from build123d import *

# Parameters (mm, degrees)
F0_W     = 50.8
F0_H     = 38.1
F1_DEPTH = 31.75
F3_DEPTH = 50.8
F4_W     = 18.9170949161
F4_H     = 6.0472670011
F4_W_2   = 4.9618594348
F5_DEPTH = 19.05
F6_DEPTH = 25.4


with BuildPart() as f1:
    # F0 (on Front) → F1 (new body)
    with BuildSketch(Plane.XZ):
        with Locations((-6.0472674668, 14.0159087854)):
            Rectangle(F0_W, F0_H)
    extrude(amount=F1_DEPTH)

    # F2 (on face) → F3 (cut)
    with BuildSketch(Plane.YZ.offset(19.3527325332)):
        with BuildLine():
            Line((-31.75, 33.0659087854), (-31.75, 6.0472674668))
            ThreePointArc((-31.75, 6.0472674668), (-11.6942038752, 12.7030410182), (-6.0472670011, 33.0659087854))
            Line((-6.0472670011, 33.0659087854), (-31.75, 33.0659087854))
        make_face()
    extrude(amount=-F3_DEPTH, mode=Mode.SUBTRACT)

    # F4 (on face) → F5 (cut)
    with BuildSketch(Plane.XY.offset(33.0659087854)):
        with Locations((-3.4112781286, -3.0236335006)):
            Rectangle(F4_W, F4_H)
        with Locations((-15.3507553041, -3.0236335006)):
            Rectangle(F4_W_2, F4_H)
    extrude(amount=-F5_DEPTH, mode=Mode.SUBTRACT)

    # F6 (cut): a face of the model
    f6_faces = [f1.faces().sort_by_distance(p)[0] for p in [
        (-5.892207846, -6.0472670011, 18.653876051),
    ]]
    extrude(f6_faces, amount=-F6_DEPTH, mode=Mode.SUBTRACT)


solid = f1.part
Can you work these out from the model? Positions are in its coordinate system, mm. A direction names the side the tool comes from. Coordinates: 2 decimals unless noted, no trailing zeros. Write each loop counter-clockwise with the first axis right and the second up, starting at its lowest first coordinate (ties: lowest second). Pieces come first, ordered by that corner, then holes. Notation, with made-up numbers: M 68.5,41 L 82.5,41 A29 ccw 82.5,72 Z; hole C -23,16.5 d5. An arc over 180 degrees is marked long. Use one line per item in the form item = value.
Q1. If we section it at A-A (z = 28): Write out the boundary of the cut face in (x, y).
Model answer:
outline = M -31.45,-5.51 L -17.83,-5.51 L -17.83,0 L -31.45,0 Z; M 6.05,-5.51 L 19.35,-5.51 L 19.35,0 L 6.05,0 Z
Q2. We'd pull the mould along X, two halves only. Please class faces 3 (the flat face through (-31.447, -12, 5)), 4 (the flat face through (-17.832, -3, 24)), 5 (the flat face through (19.353, -12, 5)), 6 (the flat face through (-6, -5, 14.016)): +X half, -X half, draft (parallel to the pull), parting line (faces both ways), or undercut.
Model answer:
face_3 = -X half
face_4 = undercut
face_5 = +X half
face_6 = undercut
Q3. For faces 1 (the flat face through (-6, 0, 10)), 2 (the flat face through (6.047, -3, 24)), which set-ups out of +Z, -Z, +X, -X, +Y, -Y let a thin tool reach every point of the face, with its end or its side?
Model answer:
face_1 = +Z, -Z, +X, -X, +Y
face_2 = +Z, +Y, -Y
Q4. I need wall thicknesses on line 1 along X through (y, z) = (-6.5, 17.5); line 2 along Z through (x, y) = (-13, -7); line 3 along Z through (x, y) = (6, -27). Which ranges of each line are inside material? Lowest first, please. Write a range as from..to.
Model answer:
line_1 = -31.45..-17.83, 6.05..19.35
line_2 = -5.03..14.02
line_3 = -5.03..5.75
Q5. If we section it at C-C (x = -21): Write out the boundary of the cut face in (y, z).
Model answer:
outline = M -31.75,-5.03 L 0,-5.03 L 0,33.07 L -6.05,33.07 A22.45 cw -31.75,6.05 Z
Q6. For P1, Ø2, axis at x = -20, z = 27, coming from the -Y side; P2, Ø5.5, axis at x = -5, y = -5.5, coming from the +Z side, each with a flat end and sliding along its axis, tell me the tip position at first contact or that it passes through.
Model answer:
P1 = -5.61
P2 = 14.02
Q7. If we section it at B-B (y = -4.5): Write out the boundary of the cut face in (x, z).
Model answer:
outline = M -31.45,-5.03 L 19.35,-5.03 L 19.35,33.07 L 6.05,33.07 L 6.05,14.02 L -17.83,14.02 L -17.83,33.07 L -31.45,33.07 Z
Q8. If we section it at D-D (y = -9.5): Write out the boundary of the cut face in (x, z), then the cut area to 3 significant figures.
Model answer:
outline = M -31.45,-5.03 L 19.35,-5.03 L 19.35,15.4 L 6.05,15.4 L 6.05,14.02 L -17.83,14.02 L -17.83,15.4 L -31.45,15.4 Z
area = 1,010 mm^2
